Geometry check sheet. Reference: the model listing, model coordinates, mm. Face numbers are marked on the shaded views. A direction names the side the tool comes from. Round coordinates to 2 decimals unless told otherwise and drop trailing zeros. Write each loop counter-clockwise with the first axis right and the second up, starting at its lowest first coordinate (ties: lowest second). Pieces come first, ordered by that corner, then holes. Notation, with made-up numbers: (76.25, 77) - (93.25, 77) arc R21 ccw to (93.25, 114) - close; hole circle Ø8 at (-15, 41). An arc over 180 degrees is marked (long way). Return JSON: item names as keys, results as strings.
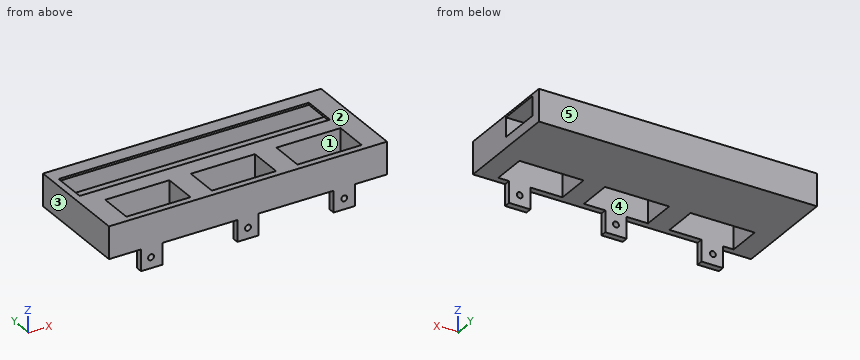
```python
from build123d import *

# Parameters (mm, degrees)
SKETCH1_W               = 130
SKETCH1_H               = 50
BOSS_EXTRUDE1_DEPTH     = 15
CUT_EXTRUDE1_DEPTH      = 185.458667457
CUT_EXTRUDE1_DEPTH_BACK = 127
SKETCH4_W               = 10
SKETCH4_H               = 3
BOSS_EXTRUDE2_DEPTH     = 10
SKETCH6_W               = 30
SKETCH6_H               = 16
CUT_EXTRUDE2_DEPTH      = 253.419918463
SKETCH7_R               = 1.375
CUT_EXTRUDE3_DEPTH      = 222.415481023
SKETCH9_W               = 10
SKETCH9_H               = 3
BOSS_EXTRUDE4_DEPTH     = 10
SKETCH10_R              = 1.375
CUT_EXTRUDE4_DEPTH      = 10
SKETCH11_W              = 10
SKETCH11_H              = 1
BOSS_EXTRUDE5_DEPTH     = 20


with BuildPart() as part:
    # Sketch1 → Boss-Extrude1 (new body)
    with BuildSketch(Plane.XY):
        with Locations((-150.849056604, 105)):
            Rectangle(SKETCH1_W, SKETCH1_H)
    extrude(amount=BOSS_EXTRUDE1_DEPTH)

    # Sketch3 → Cut-Extrude1 (cut, two sides: drawn at the far end of the back side and taken through both)
    with BuildSketch(Plane(origin=(-85.849056604, 0, 0), x_dir=(0, 0, -1), z_dir=(1, 0, 0)).offset(-CUT_EXTRUDE1_DEPTH_BACK)):
        Polygon((-14, 125), (-5, 125), (-5, 105), (-14, 105), (-14, 107), (-15, 107), (-15, 123), (-14, 123), align=None)
    extrude(amount=CUT_EXTRUDE1_DEPTH + CUT_EXTRUDE1_DEPTH_BACK, mode=Mode.SUBTRACT)

    # Sketch4 → Boss-Extrude2 (add)
    with BuildSketch(Plane(origin=(0, 0, 0), x_dir=(-1, 0, 0), z_dir=(0, 0, -1))):
        with Locations((105.849056604, 81.5)):
            Rectangle(SKETCH4_W, SKETCH4_H)
        with Locations((195.849056604, 81.5)):
            Rectangle(SKETCH4_W, SKETCH4_H)
    extrude(amount=BOSS_EXTRUDE2_DEPTH)

    # Sketch6 → Cut-Extrude2 (cut, through all)
    with BuildSketch(Plane(origin=(0, 0, 0), x_dir=(-1, 0, 0), z_dir=(0, 0, -1))):
        with Locations((190.849056604, 91)):
            Rectangle(SKETCH6_W, SKETCH6_H)
        with Locations((150.849056604, 91)):
            Rectangle(SKETCH6_W, SKETCH6_H)
        with Locations((110.849056604, 91)):
            Rectangle(SKETCH6_W, SKETCH6_H)
    extrude(amount=-CUT_EXTRUDE2_DEPTH, mode=Mode.SUBTRACT)

    # Sketch7 → Cut-Extrude3 (cut, through all)
    with BuildSketch(Plane(origin=(0, 83, 0), x_dir=(1, 0, 0), z_dir=(0, 1, 0))):
        with Locations(Location((-105.849056604, 5, 0), (0, 0, 270))):
            Circle(SKETCH7_R)
    cut_extrude3 = extrude(amount=-CUT_EXTRUDE3_DEPTH, mode=Mode.SUBTRACT)

    # Mirror1: Cut-Extrude3 across plane
    add(cut_extrude3.mirror(Plane(origin=(-151, 0, 0), x_dir=(0, 0, 1), z_dir=(1, 0, 0))), mode=Mode.SUBTRACT)

    # Sketch9 → Boss-Extrude4 (add)
    with BuildSketch(Plane(origin=(0, 0, 0), x_dir=(-1, 0, 0), z_dir=(0, 0, -1))):
        with Locations((150.849056604, 81.5)):
            Rectangle(SKETCH9_W, SKETCH9_H)
    extrude(amount=BOSS_EXTRUDE4_DEPTH)

    # Sketch10 → Cut-Extrude4 (cut)
    with BuildSketch(Plane(origin=(0, 83, 0), x_dir=(1, 0, 0), z_dir=(0, 1, 0))):
        with Locations(Location((-150.849056604, 5, 0), (0, 0, 180))):
            Circle(SKETCH10_R)
    extrude(amount=-CUT_EXTRUDE4_DEPTH, mode=Mode.SUBTRACT)

    # Sketch11 → Boss-Extrude5 (add)
    with BuildSketch(Plane(origin=(0, 107, 0), x_dir=(1, 0, 0), z_dir=(0, 1, 0))):
        with Locations((-90.849056604, -14.5)):
            Rectangle(SKETCH11_W, SKETCH11_H)
    extrude(amount=BOSS_EXTRUDE5_DEPTH)


solid = part.part
```
(1) Section check D-D, the plane z = 11.75. Enter the section's corners in (x, y), plus the area to 3 significant figures.
Response values:
{"outline": "(-215.85, 80) - (-85.85, 80) - (-85.85, 105) - (-212.85, 105) - (-212.85, 125) - (-85.85, 125) - (-85.85, 130) - (-215.85, 130) - close; hole (-205.85, 83) - (-175.85, 83) - (-175.85, 99) - (-205.85, 99) - close; hole (-165.85, 83) - (-135.85, 83) - (-135.85, 99) - (-165.85, 99) - close; hole (-125.85, 83) - (-95.85, 83) - (-95.85, 99) - (-125.85, 99) - close", "area": "2,520 mm^2"}
(2) Access from +Z, -Z, +X, -X, +Y, -Y to the whole of each face (thin tool, end or side, straight path). Record for the marked faces 4 and 5.
Response values:
{"face 4": "+Z, -Z", "face 5": "+Z, -Z, +X, -X, +Y"}
(3) Section check A-A, the plane z = -1.25. Enter the section's corners in (x, y), plus the area to 3 significant figures.
Response values:
{"outline": "(-200.85, 80) - (-190.85, 80) - (-190.85, 83) - (-200.85, 83) - close; (-155.85, 80) - (-145.85, 80) - (-145.85, 83) - (-155.85, 83) - close; (-110.85, 80) - (-100.85, 80) - (-100.85, 83) - (-110.85, 83) - close", "area": "90.0 mm^2"}
(4) Section check C-C, the plane y = 112. Enter the section's corners in (x, z), plus the area to 3 significant figures.
Response values:
{"outline": "(-215.85, 0) - (-85.85, 0) - (-85.85, 5) - (-212.85, 5) - (-212.85, 15) - (-215.85, 15) - close; (-95.85, 14) - (-85.85, 14) - (-85.85, 15) - (-95.85, 15) - close", "area": "690 mm^2"}
(5) Material ranges on line 1 along X through (y, z) = (97, 4); line 2 along Y through (x, z) = (-99.5, 7.5); line 3 along Y through (x, z) = (-204, 1.5), recorded low to high. Write a range as [from, to].
Response values:
{"line 1": "x = [-215.85, -205.85], [-175.85, -165.85], [-135.85, -125.85], [-95.85, -85.85]", "line 2": "y = [80, 83], [99, 105], [125, 130]", "line 3": "y = [80, 83], [99, 130]"}
(6) Section check B-B, the plane y = 85. Enter the section's corners in (x, z).
Response values:
{"outline": "(-215.85, 0) - (-205.85, 0) - (-205.85, 15) - (-215.85, 15) - close; (-175.85, 0) - (-165.85, 0) - (-165.85, 15) - (-175.85, 15) - close; (-135.85, 0) - (-125.85, 0) - (-125.85, 15) - (-135.85, 15) - close; (-95.85, 0) - (-85.85, 0) - (-85.85, 15) - (-95.85, 15) - close"}
(7) Gauge pin test, flat ends, axial feed: pin 1 (2.5 mm diameter, centred on y = 81.5, z = -6, fed in from -X); pin 2 (3 mm diameter, centred on y = 116.5, z = 9.5, fed in from +X); pin 3 (6 mm diameter, centred on x = -121.5, y = 117.5, fed in from +Z); pin 4 (8 mm diameter, centred on x = -143, z = -1.5, fed in from -Y). Record the tip position at first contact, or that the pin passes through.
Response values:
{"pin 1": "stops at x = -200.85", "pin 2": "stops at x = -212.85", "pin 3": "stops at z = 5", "pin 4": "stops at y = 80"}
(8) Release check for a two-part mould opening along X. For the marked faces 1, 2 and 3 record: pulls with the +X half, pulls with the -X half, needs draft (parallel to the pull), parting line crosses it, or undercut.
Response values:
{"face 1": "undercut", "face 2": "needs draft", "face 3": "pulls with the -X half"}
